Drawing for the job (mm, zero at the part's lowest x, y, z). A direction names the side the tool comes from. Coordinates: 2 decimals unless noted, no trailing zeros. Write each loop counter-clockwise with the first axis right and the second up, starting at its lowest first coordinate (ties: lowest second). Pieces come first, ordered by that corner, then holes. Notation, with made-up numbers: (9, -25) -> (68, -25) arc R17 ccw to (68, 6) -> close; hole circle Ø6 at (2, -19). An arc over 180 degrees is marked (long way). Write item = value, one per line. Start each with the question number.
Q1. Tool access for the marked faces 4, 5 and 6: list every direction of +Z, -Z, +X, -X, +Y, -Y with a clear straight run to the whole face (end or side of a thin tool).
Q2. Band-saw the part on A-A, the plane x = 67.5. List the corners of the cut face in (y, z).
Q3. Band-saw the part on B-B, the plane z = 72.5. List the corners of the cut face in (x, y), plus the area to 3 significant figures.
Q4. Pin check, flat tips, straight feed: P1, Ø7, axis at x = 8, z = 27.5, coming from the +Y side; P2, Ø2, axis at x = 74.5, z = 75, coming from the +Y side; P3, Ø8, axis at y = 62, z = 71.5, coming from the +X side. Stop position of each tip, or through.
Q5. Probe line 1 (X direction, y = 95, z = 58); line 2 (X direction, y = 23.5, z = 23); line 3 (Y direction, x = 10.5, z = 25.5). List the from-to ranges inside material, lowest first.
Q6. Band-saw the part on C-C, the plane y = 95. List the corners of the cut face in (x, z).
Q7. Band-saw the part on D-D, the plane z = 45. List the corners of the cut face in (x, y), plus the area to 3 significant figures.
Q8. Pull direction Y, two halves, no side cores. Call the marked faces 1, 2 and 3: released by +Y, released by -Y, zero draft, split by the parting line, or undercut.
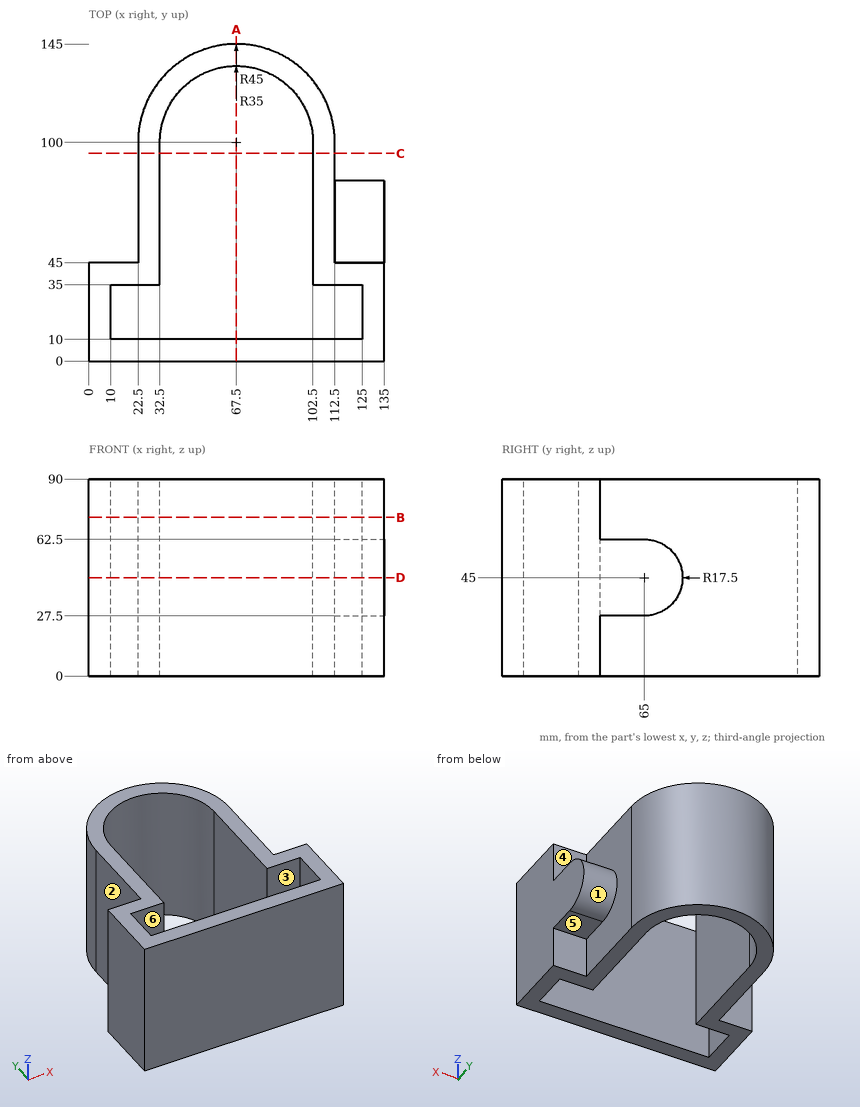
Ans:
q1.face_4 = +Z, +X, +Y
q1.face_5 = -Z, +X, +Y
q1.face_6 = +Z, -Z
q2.outline = (0, 0) -> (10, 0) -> (10, 90) -> (0, 90) -> close; (135, 0) -> (145, 0) -> (145, 90) -> (135, 90) -> close
q3.outline = (0, 0) -> (135, 0) -> (135, 45) -> (112.5, 45) -> (112.5, 100) arc R45 ccw to (22.5, 100) -> (22.5, 45) -> (0, 45) -> close; hole (10, 10) -> (125, 10) -> (125, 35) -> (102.5, 35) -> (102.5, 100) arc R35 ccw to (32.5, 100) -> (32.5, 35) -> (10, 35) -> close
q3.area = 4,860 mm2
q4.P1 = 45
q4.P2 = 144.6
q4.P3 = 112.5
q5.line_1 = 22.5 to 32.5, 102.5 to 112.5
q5.line_2 = 0 to 10, 125 to 135
q5.line_3 = 0 to 10, 35 to 45
q6.outline = (22.5, 0) -> (32.5, 0) -> (32.5, 90) -> (22.5, 90) -> close; (102.5, 0) -> (112.5, 0) -> (112.5, 90) -> (102.5, 90) -> close
q7.outline = (0, 0) -> (135, 0) -> (135, 82.5) -> (112.5, 82.5) -> (112.5, 100) arc R45 ccw to (22.5, 100) -> (22.5, 45) -> (0, 45) -> close; hole (10, 10) -> (125, 10) -> (125, 35) -> (102.5, 35) -> (102.5, 100) arc R35 ccw to (32.5, 100) -> (32.5, 35) -> (10, 35) -> close
q7.area = 5,700 mm2
q8.face_1 = released by +Y
q8.face_2 = zero draft
q8.face_3 = undercut
